```python
from build123d import *

# Parameters (mm, degrees)
F1_DEPTH = 8
F3_DEPTH = 4
F4_R     = 2.25
F5_DEPTH = 25


with BuildPart() as f1:
    # F0 (on Top) → F1 (new body)
    with BuildSketch(Plane.XY):
        Polygon((0, 24.041631), (0, 0), (7.7, 7.7), (7.7, 31.741631), align=None)
    extrude(amount=F1_DEPTH)

    # F2 (on face) → F3 (cut)
    with BuildSketch(Plane.XY.offset(8)):
        Polygon((3.75, 12.435577), (7.3, 14.485171), (7.3, 18.584358), (3.75, 20.633951), (0.2, 18.584358), (0.2, 14.485171), align=None)
    extrude(amount=-F3_DEPTH, mode=Mode.SUBTRACT)

    # F4 (on face) → F5 (cut)
    with BuildSketch(Plane.XY.offset(4)):
        with Locations((3.8, 16.534764)):
            Circle(F4_R)
    extrude(amount=-F5_DEPTH, mode=Mode.SUBTRACT)


solid = f1.part
```
Verification items for the finished model (mm, model axes). A direction names the side the tool comes from. Round coordinates to 2 decimals unless told otherwise and drop trailing zeros. Order: outer loops, then holes, each group sorted by start corner. A loop starts at its lowest first (then second) coordinate and runs counter-clockwise, first axis right, second up.
1) Cross-section at C-C, the plane y = 18. Record the cut outline in (x, z), plus the area to 3 significant figures.
Geometry says:
outline: (0, 0) - (2.09, 0) - (2.09, 4) - (0.2, 4) - (0.2, 8) - (0, 8) - close; (5.51, 0) - (7.7, 0) - (7.7, 8) - (7.3, 8) - (7.3, 4) - (5.51, 4) - close
area: 19.5 mm2
2) Tool access check on faces 5 (the flat face through (2.1, 14.8, 4)), 6 (the flat face through (3.904, 27.946, 3.944)). Record the directions out of +Z, -Z, +X, -X, +Y, -Y that give a thin tool (end or side, any length) a straight path to the whole face; none if there is none.
Geometry says:
face 5: +Z
face 6: +Z, -Z, -X, +Y
3) Draft check along Y on faces 1 (the flat face through (1.95, 13.475, 6.028)), 2 (the flat face through (0.2, 17, 6)), 3 (the flat face through (4, 4, 4)), 4 (the flat face through (7.7, 20, 4)). Enter one of: +Y half, -Y half, draft (parallel to the pull), parting line (faces both ways), or undercut.
Geometry says:
face 1: undercut
face 2: undercut
face 3: -Y half
face 4: draft
4) Depth check by flat-ended pin: pin 1 (3 mm diameter, centred on x = 3, z = 6, fed in from +Y); pin 2 (3.5 mm diameter, centred on x = 4, y = 15.5, fed in from +Z); pin 3 (1 mm diameter, centred on x = 6, z = 3.5, fed in from -Y). Enter the tip coordinate at first touch or a pass-through.
Geometry says:
pin 1: stops at y = 28.54
pin 2: stops at z = 4
pin 3: stops at y = 5.5
5) Material ranges on line 1 (X direction, y = 16.5, z = 6.25); line 2 (Y direction, x = 5.75, z = 1); line 3 (Y direction, x = 3.5, z = 1.5), recorded low to high.
Geometry says:
line 1: x = 0 to 0.2, 7.3 to 7.7
line 2: y = 5.75 to 15.41, 17.66 to 29.79
line 3: y = 3.5 to 14.3, 18.76 to 27.54
6) Cross-section at B-B, the plane x = 5. Record the cut outline in (y, z).
Geometry says:
outline: (5, 0) - (14.63, 0) - (14.63, 4) - (13.16, 4) - (13.16, 8) - (5, 8) - close; (18.44, 0) - (29.04, 0) - (29.04, 8) - (19.91, 8) - (19.91, 4) - (18.44, 4) - close
7) Cross-section at A-A, the plane z = 5.25. Record the cut outline in (x, y).
Geometry says:
outline: (0, 0) - (7.7, 7.7) - (7.7, 31.74) - (0, 24.04) - close; hole (0.2, 14.49) - (3.75, 12.44) - (7.3, 14.49) - (7.3, 18.58) - (3.75, 20.63) - (0.2, 18.58) - close
8) Cross-section at D-D, the plane x = 6.75. Record the cut outline in (y, z), plus the area to 3 significant figures.
Geometry says:
outline: (6.75, 0) - (30.79, 0) - (30.79, 8) - (18.9, 8) - (18.9, 4) - (14.17, 4) - (14.17, 8) - (6.75, 8) - close
area: 173 mm2
